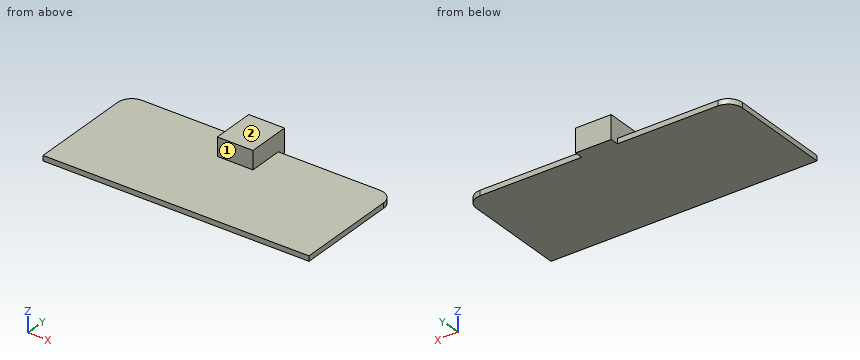
Autodesk Inventor part; units mm, degrees
ref_plane "YZ Plane" through (0, 0, 0) normal (1, 0, 0) x (0, 1, 0)
ref_plane "XZ Plane" through (0, 0, 0) normal (0, 1, 0) x (-1, 0, 0)
ref_plane "XY Plane" through (0, 0, 0) normal (0, 0, 1) x (1, 0, 0)
sketch "Sketch1: PCB" plane through (0, 0, 0) normal (0, 0, 1) x (1, 0, 0)
  line L0 (-22.0554, 53.3935) -> (34.5446, 53.3935)
  line L1 (34.5446, 53.3935) -> (34.5446, 28.5935)
  line L2 (34.5446, 28.5935) -> (-22.0554, 28.5935)
  line L3 (-22.0554, 28.5935) -> (-22.0554, 53.3935)
  line L4 (2.3446, 55.1935) -> (9.9446, 55.1935)
  line L5 (9.9446, 55.1935) -> (9.9446, 45.9935)
  line L6 (9.9446, 45.9935) -> (2.3446, 45.9935)
  line L7 (2.3446, 45.9935) -> (2.3446, 55.1935)
  point P0 (0, 0)
  dimension "d0" = 56.6
  dimension "d1" = 24.8
  dimension "d2" = 7.6
  dimension "d4" = 9.2
  dimension "d7" = 1.8
  dimension "d13" = 32
extrude "Extrusion1" add sketch "Sketch1: PCB" along normal blind 1.1 contours L0 L7 L6 L5 L1 L2 L3 | L0 L5 L6 L7
extrude "Extrusion2" add sketch "Sketch1: PCB" along normal blind 5 contours L7 L4 L5 L0 | L0 L5 L6 L7
fillet "Fillet1" radius 3 2 edges at (-22.0554, 53.3935, 0.55) (34.5446, 53.3935, 0.55)
properties part number "PCB"
For this review, take the finished solid that the model builds, in its own axes (mm). Face numbers are marked on the shaded views. A direction names the side the tool comes from. Round coordinates to 2 decimals unless told otherwise and drop trailing zeros. Order: outer loops, then holes, each group sorted by start corner. A loop starts at its lowest first (then second) coordinate and runs counter-clockwise, first axis right, second up. Notation, with made-up numbers: M 30.25,59 L 78.25,59 A19 ccw 78.25,83 Z; hole C 45,60 d2. An arc over 180 degrees is marked long. Write each question's results on one line, items separated by ' | '. Start each with the question number.
1. Add section B-B (x = 7). State the section outline as (y, z) points.
2. Add section D-D (y = 44). State the section outline as (x, z) points, then the cut area to 3 significant figures.
3. Add section A-A (y = 48.25). State the section outline as (x, z) points.
4. Clearance check with flat-ended pins moving along their axes: pin 1 Ø1.5 at (y, z) = (51.5, 3) entering from +X; pin 2 Ø1.5 at (x, y) = (-15, 47.5) entering from +Z; pin 3 Ø1.5 at (y, z) = (50.5, 3) entering from -X. State where each tip first meets the part, or that it passes through.
5. Add section C-C (z = 2.1). State the section outline as (x, y) points, then the cut area to 3 significant figures.
6. Tool access review of the marked faces 1 and 2: name each direction out of +Z, -Z, +X, -X, +Y, -Y from which nothing blocks a thin tool from reaching the whole face with its end or side.
7. To check wall thickness, follow L1, parallel to Y at x = 4, z = 2.75; L2, parallel to Z at x = -7, y = 44.5; L3, parallel to Y at x = 31.5, z = 0.85. State the ranges of each line that lie inside material, in increasing order. Write a range as [from, to].
Output values:
1) outline: M 28.59,0 L 55.19,0 L 55.19,5 L 45.99,5 L 45.99,1.1 L 28.59,1.1 Z
2) outline: M -22.06,0 L 34.54,0 L 34.54,1.1 L -22.06,1.1 Z | area: 62.3 mm^2
3) outline: M -22.06,0 L 34.54,0 L 34.54,1.1 L 9.94,1.1 L 9.94,5 L 2.34,5 L 2.34,1.1 L -22.06,1.1 Z
4) pin 1: x = 9.94 | pin 2: z = 1.1 | pin 3: x = 2.34
5) outline: M 2.34,45.99 L 9.94,45.99 L 9.94,55.19 L 2.34,55.19 Z | area: 69.9 mm^2
6) face 1: +Z, +X, -X, -Y | face 2: +Z, +X, -X, +Y, -Y
7) L1: [45.99, 55.19] | L2: [0, 1.1] | L3: [28.59, 53.39]
